Here's how the part is built. I have some questions about the finished solid (model axes, mm). A direction names the side the tool comes from. Coordinates: 2 decimals unless noted, no trailing zeros. Write each loop counter-clockwise with the first axis right and the second up, starting at its lowest first coordinate (ties: lowest second). Pieces come first, ordered by that corner, then holes. Notation, with made-up numbers: (71.25, 17) -> (129.25, 17) arc R17 ccw to (129.25, 49) -> close; hole circle Ø1 at (-31, 70). An arc over 180 degrees is marked (long way). Use a Markdown table: item, result. Add a question column.
Item 1: If we mould it in two halves opening along X, with no side actions, what happens to faces 4 (the cylindrical face through (9.539, -14.788, -1.479)), 5 (the flat face through (-10, -0.176, 10)), 6 (the cylindrical face through (11.7, -21.84, -1.48)), 7 (the cylindrical face through (0.04, 7.46, -1.48))? For each: pulls with the +X half, pulls with the -X half, needs draft (parallel to the pull), parting line crosses it, or undercut.
Item 2: Imagine slicing it at A-A, the plane z = 17. Write out the boundary of the cut face in (x, y).
Item 3: Imagine slicing it at D-D, the plane x = 5. Write out the boundary of the cut face in (y, z), and give its area (3 significant figures).
Item 4: Imagine slicing it at B-B, the plane x = -11. Write out the boundary of the cut face in (y, z).
Item 5: Imagine slicing it at C-C, the plane y = 11.5. Write out the boundary of the cut face in (x, z), and give its area (3 significant figures).
Item 6: On a 3-axis mill with a long thin cutter (end or side, diameter ignored), from which of +Z, -Z, +X, -X, +Y, -Y can I reach the whole of each face in a straight line? I mean faces 1 (the cylindrical face through (-5.352, 7.585, 18.983)), 2 (the flat face through (-4.654, 8, 18)), 3 (the cylindrical face through (-9.724, 7.541, 16.024)). Say none if no direction works.
Item 7: If I drill on line 1 along Z through (x, y) = (4, 11); line 2 along Y through (x, z) = (-12, 12.25); line 3 along X through (y, z) = (-15.5, -0.5), over which ranges is the centre line in solid material (lowest first)? Write a range as from..to.
Item 8: Will these pins go through, and if not, where does the flat tip stop? pin 1 Ø2.5 at (y, z) = (7.32, 17) entering from -X; pin 2 Ø12 at (x, z) = (-10.5, 10) entering from -Y; pin 3 Ø15.5 at (x, y) = (4.5, -10) entering from +Z; pin 4 Ø1.2 at (y, z) = (7.5, 18) entering from +X.
```python
from build123d import *

# Parameters (mm, degrees)
F0_R     = 1.4
F0_W     = 10
F0_H     = 15
F3_DEPTH = 3
F2_W     = 8
F2_H     = 15
F5_R     = 2
F5_R_2   = 1
F6_DEPTH = 10
F7_DEPTH = 15
F8_R     = 1


with BuildPart() as f3:
    # F0 (on Top) → F3 (new body)
    with BuildSketch(Plane.XY):
        with BuildLine():
            Line((-2.3220218662, -1.1490219488), (4.1030128133, -18.2824477607))
            ThreePointArc((4.1030128133, -18.2824477607), (11.8277285282, -21.7936821766), (15.3389629441, -14.0689664616))
            Line((15.3389629441, -14.0689664616), (5.9639629441, 10.9310335384))
            ThreePointArc((5.9639629441, 10.9310335384), (3.7635569052, 13.7558465942), (0.3459878787, 14.8242928889))
            Line((0.3459878787, 14.8242928889), (-4.6540121213, 14.8242928889))
            Line((-4.6540121213, 14.8242928889), (-4.6540121213, -0.1757071111))
            Line((-4.6540121213, -0.1757071111), (-3.7265156326, -0.1757071111))
            ThreePointArc((-3.7265156326, -0.1757071111), (-2.8721233759, -0.4428186848), (-2.3220218662, -1.1490219488))
        make_face()
        with Locations((9.7209878787, -16.1757071111)):
            Circle(F0_R, mode=Mode.SUBTRACT)
        with Locations((0.3459878787, 8.8242928889)):
            Circle(F0_R, mode=Mode.SUBTRACT)
        with Locations((-9.6540121213, 7.3242928889)):
            Rectangle(F0_W, F0_H)
    extrude(amount=-F3_DEPTH)

    # F0 (on Top) → F4 section 0
    with BuildSketch(Plane.XY):
        with Locations((-9.6540121213, 7.3242928889)):
            Rectangle(F0_W, F0_H)
    # F2 (on offset) → F4 section 1
    with BuildSketch(Plane.XY.offset(22)):
        with Locations((-10.6540121213, 7.3242928889)):
            Rectangle(F2_W, F2_H)
    loft()

    # F5 (on face) → F6 (join)
    with BuildSketch(Plane(origin=(-14.6540121213, 0, 0), x_dir=(0, -1, 0), z_dir=(-1, 0, 0))):
        with Locations((-7.3242928889, 17)):
            Circle(F5_R)
        with Locations((-7.3242928889, 17)):
            Circle(F5_R_2, mode=Mode.SUBTRACT)
    extrude(amount=-F6_DEPTH)

    # F5 (on face) → F7 (cut)
    with BuildSketch(Plane(origin=(-14.6540121213, 0, 0), x_dir=(0, -1, 0), z_dir=(-1, 0, 0))):
        with Locations((-7.3242928889, 17)):
            Circle(F5_R_2)
    extrude(amount=-F7_DEPTH, mode=Mode.SUBTRACT)

    # F8
    f8_edges = [f3.edges().sort_by_distance(p)[0] for p in [
        (-6.654012, 7.324293, 22),
        (-4.654012, 7.324293, 0),
        (-14.654012, 7.324293, 22),
    ]]
    fillet(f8_edges, radius=F8_R)


solid = f3.part
```
Ans:
| question | item | result |
|---|---|---|
| 1 | face 4 | undercut |
| 1 | face 5 | needs draft |
| 1 | face 6 | parting line crosses it |
| 1 | face 7 | undercut |
| 2 | outline | (-14.65, -0.18) -> (-6.2, -0.18) -> (-6.2, 5.32) -> (-4.65, 5.32) -> (-4.65, 6.32) -> (-14.65, 6.32) -> close; (-14.65, 8.32) -> (-4.65, 8.32) -> (-4.65, 9.32) -> (-6.2, 9.32) -> (-6.2, 14.82) -> (-14.65, 14.82) -> close |
| 3 | outline | (-19.88, -3) -> (12.61, -3) -> (12.61, 0) -> (-19.88, 0) -> close |
| 3 | area | 97.5 mm^2 |
| 4 | outline | (-0.18, -3) -> (14.82, -3) -> (14.82, 22) -> (-0.18, 22) -> close; hole circle Ø2 at (7.32, 17) |
| 5 | outline | (-14.65, -3) -> (5.72, -3) -> (5.72, 0) -> (-3.74, 0) arc R1 cw to (-4.74, 0.91) -> (-6.57, 21.09) arc R1 ccw to (-7.57, 22) -> (-13.65, 22) arc R1 ccw to (-14.65, 21) -> close |
| 5 | area | 259 mm^2 |
| 6 | face 1 | +X |
| 6 | face 2 | +Z, +X, +Y, -Y |
| 6 | face 3 | +X, -X |
| 7 | line 1 | z = -3..0 |
| 7 | line 2 | y = -0.18..14.82 |
| 7 | line 3 | x = 3.06..8.49, 10.95..15.68 |
| 8 | pin 1 | stops at x = -14.65 |
| 8 | pin 2 | stops at y = -0.18 |
| 8 | pin 3 | stops at z = 0 |
| 8 | pin 4 | stops at x = -4.65 |
